```python
from build123d import *

# Parameters (mm, degrees)
EXTRUDE_1_DEPTH      = 1
FILLET_1_R           = 4
EXTRUDE_2_DEPTH      = 2.5
EXTRUDE_2_DEPTH_BACK = 1
CHAMFER_1_SIZE       = 2
CHAMFER_3_SIZE       = 1
CUT_EXTRUDE_1_REACH  = 28.172
SKETCH_3_R           = 0.9000000000000004


with BuildPart() as part:
    # 草图1 → 凸台-拉伸1 (new body)
    with BuildSketch(Plane(origin=(0, 0, 0), x_dir=(1, 0, 0), z_dir=(0, 1, 0))):
        Polygon((-21.300000000000004, 13.800000000000002), (21.299999999999997, 13.800000000000002), (21.3, -13.799999999999999), (-21.3, -13.799999999999999), align=None)
    extrude(amount=EXTRUDE_1_DEPTH)

    # 圆角1
    fillet_1_edges = [part.edges().sort_by_distance(p)[0] for p in [
        (21.3, 0.5, 13.799999999999999),
        (-21.3, 0.5, 13.799999999999999),
        (-21.300000000000004, 0.5, -13.800000000000002),
        (21.299999999999997, 0.5, -13.800000000000002),
    ]]
    fillet(fillet_1_edges, radius=FILLET_1_R)

    # 草图2 → 凸台-拉伸2 (add, two sides: drawn at the far end of the back side and taken through both)
    with BuildSketch(Plane(origin=(0, 1, 0), x_dir=(1, 0, 0), z_dir=(0, 1, 0)).offset(-EXTRUDE_2_DEPTH_BACK)):
        Polygon((17.4, -13.800000000000002), (16.208246407405806, -14.8), (-16.208246407405806, -14.8), (-17.4, -13.800000000000002), align=None)
        Polygon((-17.400000000000002, 13.799999999999994), (-16.208246407405802, 14.8), (16.208246407405802, 14.8), (17.400000000000002, 13.799999999999994), align=None)
    extrude(amount=EXTRUDE_2_DEPTH + EXTRUDE_2_DEPTH_BACK)

    # 倒角1
    chamfer_1_edges = [part.edges().sort_by_distance(p)[0] for p in [
        (0, 0, 14.8),
        (0, 0, -14.8),
    ]]
    chamfer(chamfer_1_edges, length=CHAMFER_1_SIZE - 0.0001)  # a hair under: the kernel refuses the full size

    # 倒角3
    chamfer_3_edges = [part.edges().sort_by_distance(p)[0] for p in [
        (-3.55e-15, 1, -13.800000000000002),
        (0, 1, 13.799999999999999),
    ]]
    chamfer(chamfer_3_edges, length=CHAMFER_3_SIZE)

    # 草图3 → 切除-拉伸1 (cut, up to next)
    with BuildSketch(Plane.XZ, mode=Mode.PRIVATE) as cut_extrude_1_sk1:
        with Locations((-20.500000000000004, 4.65)):
            Circle(SKETCH_3_R)
    cut_extrude_1_tool1 = extrude(cut_extrude_1_sk1.sketch, amount=-CUT_EXTRUDE_1_REACH, mode=Mode.PRIVATE) & part.part
    # 草图3 → 切除-拉伸1 (cut, up to next)
    with BuildSketch(Plane.XZ, mode=Mode.PRIVATE) as cut_extrude_1_sk2:
        with Locations((-20.500000000000004, -4.65)):
            Circle(SKETCH_3_R)
    cut_extrude_1_tool2 = extrude(cut_extrude_1_sk2.sketch, amount=-CUT_EXTRUDE_1_REACH, mode=Mode.PRIVATE) & part.part
    # 草图3 → 切除-拉伸1 (cut, up to next)
    with BuildSketch(Plane.XZ, mode=Mode.PRIVATE) as cut_extrude_1_sk3:
        with Locations((20.50000000000001, -4.649999999999995)):
            Circle(SKETCH_3_R)
    cut_extrude_1_tool3 = extrude(cut_extrude_1_sk3.sketch, amount=-CUT_EXTRUDE_1_REACH, mode=Mode.PRIVATE) & part.part
    # 草图3 → 切除-拉伸1 (cut, up to next)
    with BuildSketch(Plane.XZ, mode=Mode.PRIVATE) as cut_extrude_1_sk4:
        with Locations((20.500000000000004, 4.650000000000006)):
            Circle(SKETCH_3_R)
    cut_extrude_1_tool4 = extrude(cut_extrude_1_sk4.sketch, amount=-CUT_EXTRUDE_1_REACH, mode=Mode.PRIVATE) & part.part
    add(cut_extrude_1_tool1.solids().sort_by_distance((-20.5, 0, 4.65))[0], mode=Mode.SUBTRACT)
    add(cut_extrude_1_tool2.solids().sort_by_distance((-20.5, 0, -4.65))[0], mode=Mode.SUBTRACT)
    add(cut_extrude_1_tool3.solids().sort_by_distance((20.5, 0, -4.65))[0], mode=Mode.SUBTRACT)
    add(cut_extrude_1_tool4.solids().sort_by_distance((20.5, 0, 4.65))[0], mode=Mode.SUBTRACT)


solid = part.part
```
Here's how the part is built. I have some questions about the finished solid (model axes, mm). A direction names the side the tool comes from. Coordinates: 2 decimals unless noted, no trailing zeros. Order: outer loops, then holes, each group sorted by start corner. A loop starts at its lowest first (then second) coordinate and runs counter-clockwise, first axis right, second up. Notation, with made-up numbers: M 7.25,-31 L 25.25,-31 A21 ccw 25.25,-9 Z; hole C 89,51 d8. An arc over 180 degrees is marked long. Answer as a JSON object with one key per item and string values. Group by question number.
(1) Suppose I cut it at B-B, the plane y = 2.45. Please give me the cut outline in (x, z).
(2) For pin 1 (1.6 mm diameter, centred on x = 20.5, z = 4.65, fed in from -Y); pin 2 (13 mm diameter, centred on x = -6, z = -0.5, fed in from +Y), each with a flat end and sliding along its axis, tell me the tip position at first contact or that it passes through.
(3) Suppose I cut it at C-C, the plane x = -8. Please give me the cut outline in (y, z), then the cut area to 3 significant figures.
(4) Suppose I cut it at A-A, the plane x = 20.5. Please give me the cut outline in (y, z), then the cut area to 3 significant figures.
(5) I need wall thicknesses on probe 1 along Z at (x, y) = (20.5, 0.5); probe 2 along Z at (x, y) = (-13.5, 2.1); probe 3 along Y at (x, z) = (-11, -10.25). Which ranges of each line are inside material? Lowest first, please.
(6) Which directions (+Z, -Z, +X, -X, +Y, -Y) give clear straight access to the entire face, cutting with the end or side of a thin tool? Please do faces 5 (the face through (0.3, 1.5, 13.3)), 6 (the face through (-16.812, 2.51, -14.293)).
(7) Suppose I cut it at D-D, the plane z = -3. Please give me the cut outline in (x, y), then the cut area to 3 significant figures.
(8) If we mould it in two halves opening along X, with no side actions, what happens to faces 1 (the face through (19.6, 0.5, 4.7)), 2 (the face through (0, 3, -14.8)), 3 (the face through (19.6, 0.5, -4.6)), 4 (the face through (-16.796, 2.51, 14.307))? For each: released by +X, released by -X, zero draft, split by the parting line, or undercut.
Values found:
{
 "1": {"outline": "M -17.4,-13.8 L -16.21,-14.8 L 16.21,-14.8 L 17.4,-13.8 Z; M -17.4,13.8 L 17.4,13.8 L 16.21,14.8 L -16.21,14.8 Z"},
 "2": {"pin 1": "passes through", "pin 2": "stops at y = 1"},
 "3": {"outline": "M 0,-12.8 L 2,-14.8 L 3.5,-14.8 L 3.5,-13.8 L 2,-13.8 L 1,-12.8 L 1,12.8 L 2,13.8 L 3.5,13.8 L 3.5,14.8 L 2,14.8 L 0,12.8 Z", "area": "31.6 mm^2"},
 "4": {"outline": "M 0,-12.2 L 1,-12.2 L 1,-5.55 L 0,-5.55 Z; M 0,-3.75 L 1,-3.75 L 1,3.75 L 0,3.75 Z; M 0,5.55 L 1,5.55 L 1,12.2 L 0,12.2 Z", "area": "20.8 mm^2"},
 "5": {"probe 1": "z = -12.2 to -5.55, -3.75 to 3.75, 5.55 to 12.2", "probe 2": "z = -14.8 to -13.8, 13.8 to 14.8", "probe 3": "y = 0 to 1"},
 "6": {"face 5": "+X, -X, +Y", "face 6": "-Z, -X, +Y, -Y"},
 "7": {"outline": "M -21.3,0 L 21.3,0 L 21.3,1 L -21.3,1 Z", "area": "42.6 mm^2"},
 "8": {"face 1": "undercut", "face 2": "zero draft", "face 3": "undercut", "face 4": "released by -X"}
}
